from build123d import *

# Parameters (mm, degrees)
SKETCH1_R           = 2
BOSS_EXTRUDE1_DEPTH = 48.26
SKETCH2_W           = 9.068360996
SKETCH2_H           = 9.379909118
BOSS_EXTRUDE2_DEPTH = 6.604
SKETCH3_W           = 9.068360996
SKETCH3_H           = 2.338852908
BOSS_EXTRUDE3_DEPTH = 12.7
SKETCH5_OUTSIDE_W   = 24.83
SKETCH5_OUTSIDE_H   = 25.142
SKETCH5_OUTSIDE_R   = 4.689954559
CUT_EXTRUDE2_DEPTH  = 68.878189152
SKETCH6_R           = 0.635
BOSS_EXTRUDE4_DEPTH = 4.702203303


# Read off the part's stored shape, not the designer's step: Mirror4
with BuildPart() as part:
    # Sketch1 → Boss-Extrude1 (new body)
    with BuildSketch(Plane.XY):
        with Locations(Location((0, 0, 0), (0, 0, 180))):
            Circle(SKETCH1_R)
    extrude(amount=BOSS_EXTRUDE1_DEPTH)

    # Sketch2 → Boss-Extrude2 (add)
    with BuildSketch(Plane.XY.offset(48.26)):
        Rectangle(SKETCH2_W, SKETCH2_H)
    extrude(amount=BOSS_EXTRUDE2_DEPTH)

    # Sketch3 → Boss-Extrude3 (add)
    with BuildSketch(Plane.XY.offset(54.864)):
        with Locations((0, 3.520528105)):
            Rectangle(SKETCH3_W, SKETCH3_H)
    boss_extrude3 = extrude(amount=BOSS_EXTRUDE3_DEPTH)

    # Mirror1: Boss-Extrude3 across plane
    add(boss_extrude3.mirror(Plane.ZX))

    # Sketch5 outside → Cut-Extrude2 (cut, through all)
    with BuildSketch(Plane.XY.offset(67.564)):
        Rectangle(SKETCH5_OUTSIDE_W, SKETCH5_OUTSIDE_H)
        Circle(SKETCH5_OUTSIDE_R, mode=Mode.SUBTRACT)
    extrude(amount=-CUT_EXTRUDE2_DEPTH, mode=Mode.SUBTRACT)

    # Sketch6 → Boss-Extrude4 (add)
    with BuildSketch(Plane(origin=(0, -2.351101651, 0), x_dir=(1, 0, 0), z_dir=(0, 1, 0))):
        with Locations(Location((0, -65.024, 0), (0, 0, 270))):
            Circle(SKETCH6_R)
    extrude(amount=BOSS_EXTRUDE4_DEPTH)

    # Mirror4: part across plane


with BuildPart() as part_1:
    add(part.part)
    add(part.part.mirror(Plane(origin=(0, 0, 0), x_dir=(1, 0, 0), z_dir=(0, 0, -1))))


solid = part_1.part
Work out the finished part from the listing and answer in its coordinate system (mm). A direction names the side the tool comes from. Give positions to 0.01 mm unless a question says otherwise; leave off trailing zeros. Order: outer loops, then holes, each group sorted by start corner. A loop starts at its lowest first (then second) coordinate and runs counter-clockwise, first axis right, second up. Notation, with made-up numbers: (83, 73) -> (103, 73) arc R18 cw to (103, 88) -> close; hole circle Ø9 at (0, 48). An arc over 180 degrees is marked (long way). Answer as a JSON object with one key per item and string values. Group by question number.
1. Flat-ended cylindrical pins translate along their axes: pin 1 Ø1.4 at (x, y) = (1, 0) entering from -Z; pin 2 Ø1.4 at (x, y) = (1.5, 0.5) entering from +Z; pin 3 Ø5 at (y, z) = (-2.5, -8) entering from -X. Find the tip coordinate at first contact, or state that the pin passes through.
2. The mould has two halves that part along Z. Classify faces 3 (the cylindrical face through (0.09, 4.69, 58.05)), 4 (the flat face through (0, -3, -67.564)), 5 (the cylindrical face through (0, 2, 1)): released by +Z, released by -Z, zero draft, split by the parting line, or undercut.
3. Consider line 1 along Z through (x, y) = (-3.75, 0.5); line 2 along Z through (x, y) = (-3.25, -2.5); line 3 along Z through (x, y) = (-1, 1.5). Determine where each line is inside the solid, lowest interval first. Write a range as [from, to].
4. A tool of negligible diameter and unlimited length cuts with its end or side. For faces 1 (the flat face through (0, 3, -67.564)), 2 (the flat face through (-0.1, 2.2, 48.26)), from which of +Z, -Z, +X, -X, +Y, -Y can it reach the whole face along a straight path? Write none if from no direction.
5. Section B-B on z = -7.5 is taken. Determine the outline of the cut face in (x, y), plus the area to 3 significant figures.
6. Section A-A on y = 0 is taken. Determine the outline of the cut face in (x, z) (3 decimals).
Result sheet:
{
 "1": {"pin 1": "stops at z = -65.58", "pin 2": "stops at z = 54.86", "pin 3": "stops at x = -2"},
 "2": {"face 3": "zero draft", "face 4": "released by -Z", "face 5": "undercut"},
 "3": {"line 1": "z = [-54.86, -48.26], [48.26, 54.86]", "line 2": "z = [-67.56, -48.26], [48.26, 67.56]", "line 3": "z = [-54.86, 54.86]"},
 "4": {"face 1": "-Z, +X, -X, +Y, -Y", "face 2": "none"},
 "5": {"outline": "circle Ø4 at (0, 0)", "area": "12.6 mm^2"},
 "6": {"outline": "(-4.534, -54.864) -> (4.534, -54.864) -> (4.534, -48.26) -> (2, -48.26) -> (2, 48.26) -> (4.534, 48.26) -> (4.534, 54.864) -> (-4.534, 54.864) -> (-4.534, 48.26) -> (-2, 48.26) -> (-2, -48.26) -> (-4.534, -48.26) -> close; circle Ø1.27 at (0, -65.024); circle Ø1.27 at (0, 65.024)"}
}
